Source: CAD feature listing. Evaluate the final solid. Frame: model axes, mm. Coordinates: 2 decimals unless noted, no trailing zeros. Loops run counter-clockwise (first coordinate to the right, second up) from the corner with the lowest first, then second, coordinate; pieces in that order, holes last. Notation, with made-up numbers: M 1.5,-13.5 L 55.5,-13.5 A25 ccw 55.5,23.5 Z; hole C 65,3.5 d5. An arc over 180 degrees is marked long. One line per question, with ' | ' between items. Start each with the question number.
1. Section query B-B, the plane y = 0. Output: boundary loops of the cut face in (x, z), and give its area (3 significant figures).
2. Section query A-A, the plane x = 0. Output: boundary loops of the cut face in (y, z), and give its area (3 significant figures).
3. Pin query (flat end, axial travel): P1, Ø1.5, axis at x = -13, z = 0.5, coming from the +Y side; P2, Ø2, axis at x = -13, z = 2, coming from the +Y side; P3, Ø3.5, axis at x = 28.194, y = 0, coming from the -Z side (3 decimals); P4, Ø1, axis at y = -9.5, z = 1.5, coming from the +X side. Return the tip coordinate at first contact, or that it passes through.
4. Section query C-C, the plane z = 3.1. Output: boundary loops of the cut face in (x, y), and give its area (3 significant figures).
5. Ray query, probe 1 along X at (y, z) = (2, 2.3) (3 decimals); probe 2 along Y at (x, z) = (-24.5, 2.7); probe 3 along X at (y, z) = (32, 0.6). Return the intervals inside material, ascending.
```python
from build123d import *

# Parameters (mm, degrees)
F0_R     = 36.5
F0_R_2   = 2.794
F1_DEPTH = 3.81
F2_SIZE  = 1.27


with BuildPart() as f1:
    # F0 (on Top) → F1 (new body)
    with BuildSketch(Plane.XY):
        Circle(F0_R)
        with Locations((-28.194, 0)):
            Circle(F0_R_2, mode=Mode.SUBTRACT)
        with Locations((28.194, 0)):
            Circle(F0_R_2, mode=Mode.SUBTRACT)
        with Locations((0, 28.194)):
            Circle(F0_R_2, mode=Mode.SUBTRACT)
    extrude(amount=F1_DEPTH)

    # F2
    f2_edges = [f1.edges().sort_by_distance(p)[0] for p in [
        (-36.5, 0, 0),
    ]]
    chamfer(f2_edges, length=F2_SIZE)


solid = f1.part
```
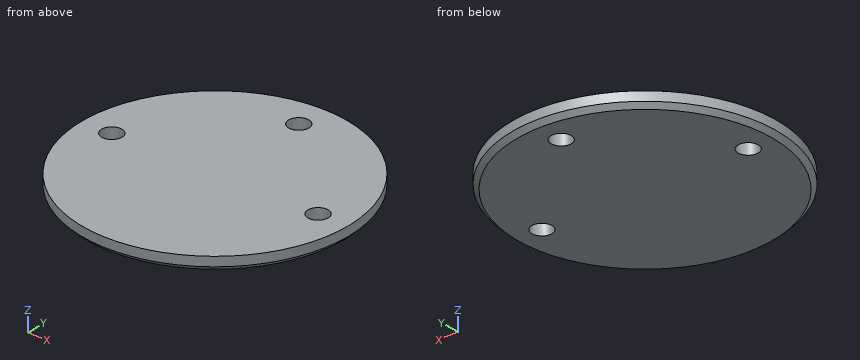
Taken from the geometry:
1) outline: M -36.5,1.27 L -35.23,0 L -30.99,0 L -30.99,3.81 L -36.5,3.81 Z; M -25.4,0 L 25.4,0 L 25.4,3.81 L -25.4,3.81 Z; M 30.99,0 L 35.23,0 L 36.5,1.27 L 36.5,3.81 L 30.99,3.81 Z | area: 234 mm^2
2) outline: M -36.5,1.27 L -35.23,0 L 25.4,0 L 25.4,3.81 L -36.5,3.81 Z; M 30.99,0 L 35.23,0 L 36.5,1.27 L 36.5,3.81 L 30.99,3.81 Z | area: 255 mm^2
3) P1: y = 34.13 | P2: y = 34.47 | P3: through | P4: x = 35.37
4) outline: C 0,0 d73; hole C -28.19,0 d5.59; hole C 0,28.19 d5.59; hole C 28.19,0 d5.59 | area: 4,110 mm^2
5) probe 1: -36.445 to -30.145, -26.243 to 26.243, 30.145 to 36.445 | probe 2: -27.06 to 27.06 | probe 3: -16.12 to 16.12
